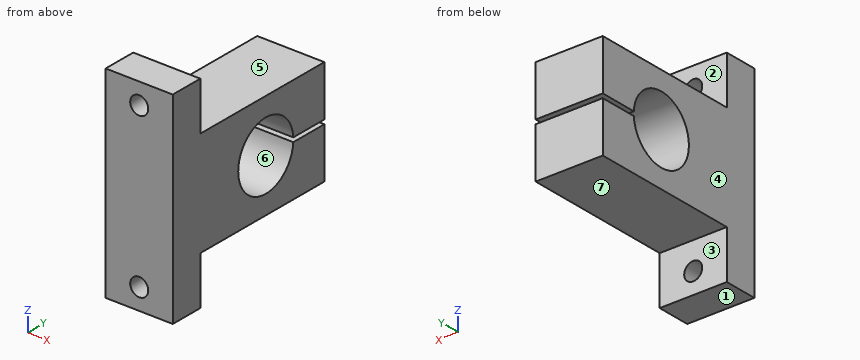
from build123d import *

# Parameters (mm, degrees)
BOSS_EXTRUDE1_DEPTH  = 16
M4_CLEARANCE_HOLE2_D = 4.3


with BuildPart() as part:
    # Sketch1 → Boss-Extrude1 (new body)
    with BuildSketch(Plane(origin=(0, 0, 0), x_dir=(0, 0, -1), z_dir=(1, 0, 0))):
        with BuildLine():
            Line((12.5, 8), (24, 8))
            Line((24, 8), (24, 0))
            Line((24, 0), (-24, 0))
            Line((-24, 0), (-24, 8))
            Line((-24, 8), (-12.5, 8))
            Line((-12.5, 8), (-12.5, 44))
            Line((-12.5, 44), (-0.5, 44))
            Line((-0.5, 44), (-0.5, 34.984359711))
            ThreePointArc((-0.5, 34.984359711), (0, 19), (0.5, 34.984359711))
            Line((0.5, 34.984359711), (0.5, 44))
            Line((0.5, 44), (12.5, 44))
            Line((12.5, 44), (12.5, 8))
        make_face()
    extrude(amount=BOSS_EXTRUDE1_DEPTH)

    # M4 Clearance Hole2 (through all)
    with Locations(Plane(origin=(0, 8, 0), x_dir=(1, 0, 0), z_dir=(0, 1, 0))):
        with Locations((8, 19), (8, -19)):
            Hole(M4_CLEARANCE_HOLE2_D / 2)


solid = part.part
The model under review builds one solid part; all positions refer to its coordinate system, in mm. Face numbers are marked on the shaded views. A direction names the side the tool comes from. Give positions to 0.01 mm unless a question says otherwise; leave off trailing zeros. Write each loop counter-clockwise with the first axis right and the second up, starting at its lowest first coordinate (ties: lowest second). Pieces come first, ordered by that corner, then holes.
1. Add section B-B, the plane x = 7.75. Write out the cut boundary in (y, z), plus the area to 3 significant figures.
2. Tool access review of the marked faces 1, 2 and 3: name each direction out of +Z, -Z, +X, -X, +Y, -Y from which nothing blocks a thin tool from reaching the whole face with its end or side.
3. For P1, Ø2.5, axis at x = 6.5, y = 38.5, coming from the +Z side; P2, Ø7, axis at x = 10.5, y = 41, coming from the -Z side; P3, Ø9, axis at x = 8.5, z = -20, coming from the +Y side; P4, Ø2.5, axis at x = 8, z = 19, coming from the -Y side, all flat-tipped, find the tip position at first contact; note any pin that passes through.
4. Wall thickness on L1, parallel to Z at x = 8, y = 6; L2, parallel to X at y = 4, z = 19; L3, parallel to Z at x = 9, y = 27: over which ranges is each line inside the solid? List them lowest first.
5. Add section C-C, the plane y = 27. Write out the cut boundary in (x, z), plus the area to 3 significant figures.
6. Add section D-D, the plane x = 4.75. Write out the cut boundary in (y, z).
7. Add section A-A, the plane z = 19. Write out the cut boundary in (x, y), plus the area to 3 significant figures.
8. Draft analysis for pull direction Z (two halves, no side actions). For the marked faces 4, 5, 6 and 7, state which applies: +Z half, -Z half, draft (parallel to the pull), parting line (faces both ways), or undercut.
Worked answers:
1. outline: (0, -24) - (8, -24) - (8, -21.14) - (0, -21.14) - close; (0, -16.86) - (8, -16.86) - (8, -12.5) - (44, -12.5) - (44, -0.5) - (34.98, -0.5) arc R8 cw (long way) to (34.98, 0.5) - (44, 0.5) - (44, 12.5) - (8, 12.5) - (8, 16.86) - (0, 16.86) - close; (0, 21.14) - (8, 21.14) - (8, 24) - (0, 24) - close
1. area: 1,010 mm2
2. face 1: -Z, +X, -X, +Y, -Y
2. face 2: +Z, +X, -X, +Y
2. face 3: -Z, +X, -X, +Y
3. P1: stops at z = 12.5
3. P2: stops at z = -12.5
3. P3: stops at y = 8
3. P4: passes through
4. L1: z = -24 to -21.15, -16.85 to 16.85, 21.15 to 24
4. L2: x = 0 to 5.85, 10.15 to 16
4. L3: z = -12.5 to -8, 8 to 12.5
5. outline: (0, -12.5) - (16, -12.5) - (16, -8) - (0, -8) - close; (0, 8) - (16, 8) - (16, 12.5) - (0, 12.5) - close
5. area: 144 mm2
6. outline: (0, -24) - (8, -24) - (8, -12.5) - (44, -12.5) - (44, -0.5) - (34.98, -0.5) arc R8 cw (long way) to (34.98, 0.5) - (44, 0.5) - (44, 12.5) - (8, 12.5) - (8, 24) - (0, 24) - close
7. outline: (0, 0) - (5.85, 0) - (5.85, 8) - (0, 8) - close; (10.15, 0) - (16, 0) - (16, 8) - (10.15, 8) - close
7. area: 93.6 mm2
8. face 4: draft
8. face 5: +Z half
8. face 6: undercut
8. face 7: -Z half
